The model under review builds one solid part; all positions refer to its coordinate system, in mm. Face numbers are marked on the shaded views. A direction names the side the tool comes from. Round coordinates to 2 decimals unless told otherwise and drop trailing zeros. Write each loop counter-clockwise with the first axis right and the second up, starting at its lowest first coordinate (ties: lowest second). Pieces come first, ordered by that corner, then holes.
Item 1: Add section B-B (z = 153). Give the boundary of the cut face in (x, y) (3 decimals), plus the area to 4 significant figures.
Item 2: Clearance check with flat-ended pins moving along their axes: pin 1 Ø1.2 at (x, z) = (4, 10) entering from +Y (3 decimals); pin 2 Ø4 at (x, z) = (-3, 182) entering from +Y (3 decimals); pin 3 Ø10 at (x, z) = (4, 85) entering from -Y (3 decimals). State where each tip first meets the part, or that it passes through.
Item 3: Add section A-A (x = 0.5). Give the boundary of the cut face in (y, z) (3 decimals), plus the area to 3 significant figures.
Item 4: To check wall thickness, follow L1, parallel to Y at x = 14.75, z = 3.5 (3 decimals); L2, parallel to Z at x = 11, y = 9.5; L3, parallel to X at y = -9.65, z = 3.5. State the ranges of each line that lie inside material, in increasing order.
Item 5: Machinability: for the marked faces 1, 2, 3, 4 and 5, which of the approach directions +Z, -Z, +X, -X, +Y, -Y give a long, thin tool a straight path to every point of the face, cutting with its end or side? Answer none if there is none.
Autodesk Inventor part; units mm, degrees
ref_plane "YZ Plane" through (0, 0, 0) normal (1, 0, 0) x (0, 1, 0)
ref_plane "XZ Plane" through (0, 0, 0) normal (0, 1, 0) x (-1, 0, 0)
ref_plane "XY Plane" through (0, 0, 0) normal (0, 0, 1) x (1, 0, 0)
sketch "Sketch8" plane through (0, 0, 0) normal (0, 0, 1) x (1, 0, 0)
  line L0 (-18.5, -12.375) -> (18.5, -12.375)
  line L1 (18.5, -12.375) -> (18.5, 12.375)
  line L2 (18.5, 12.375) -> (-18.5, 12.375)
  line L3 (-18.5, 12.375) -> (-18.5, -12.375)
  line L4 (-18.5, -12.375) -> (18.5, 12.375) construction
  line L5 (18.5, -12.375) -> (-18.5, 12.375) construction
  point P0 (0, 0)
  dimension "d43" = 37
  dimension "d44" = 24.75
extrude "Extrusion6" add sketch "Sketch8" along normal blind 7
sketch "Sketch9" plane through (0, 0, 7) normal (0, 0, 1) x (1, 0, 0)
  line L0 (-17, -10.875) -> (17, -10.875)
  line L1 (17, -10.875) -> (17, 10.875)
  line L2 (17, 10.875) -> (-17, 10.875)
  line L3 (-17, 10.875) -> (-17, -10.875)
  line L4 (-17, -10.875) -> (17, 10.875) construction
  line L5 (17, -10.875) -> (-17, 10.875) construction
  line L6 (18.5, 12.375) -> (-18.5, 12.375)
  line L7 (18.5, -12.375) -> (18.5, 12.375)
  point P0 (0, 0)
  dimension "d49" = 1.5
  dimension "d50" = 1.5
extrude "Extrusion7" add sketch "Sketch9" along normal blind 184.3
sketch "Sketch10" plane through (18.5, -12.375, 0) normal (1, 0, 0) x (0, 0, -1)
  circle A0 centre (-3.5, 21.325) radius 1.5
  line L0 (0, 0) -> (0, 24.75)
  line L1 (0, 24.75) -> (-7, 24.75)
  point P0 (0, 12.375)
  dimension "d53" = 3
  dimension "d56" = 3.425
  dimension "d57" = 3.5
hole "Hole1" at (18.5, 8.95, 3.5) direction (-1, 0, 0) diameter 3 depth 5 tip angle 118
mirror "Mirror1" about plane through (0, 0, 0) normal (0, 1, 0) of "Hole1"
mirror "Mirror2" about plane through (0, 0, 0) normal (1, 0, 0) of "Hole1", "Mirror1"
sketch "Sketch11" plane through (-18.5, -12.375, 0) normal (0, -1, 0) x (1, 0, 0)
  line L0 (18.5, 0) -> (18.5, 7)
  line L1 (37, 7) -> (0, 7)
  line L2 (18.5, 3.5) -> (0, 3.5)
  line L3 (0, 0) -> (0, 7)
  circle A0 centre (9.25, 3.5) radius 1.5
  dimension "d66" = 3
hole "Hole2" at (-9.25, -12.375, 3.5) direction (0, 1, 0) diameter 3 depth 5 tip angle 118
mirror "Mirror3" about plane through (0, 0, 0) normal (1, 0, 0) of "Hole2"
sketch "Sketch12" plane through (0, 0, 191.3) normal (0, 0, 1) x (1, 0, 0)
  circle A0 centre (6.8, 0) radius 1.5
  line L0 (17, -10.875) -> (17, 10.875)
  line L1 (17, 10.875) -> (-17, 10.875)
  point P0 (0, 0)
  dimension "d74" = 3
  dimension "d75" = 10.2
  dimension "d76" = 10.875
hole "Hole3" at (6.8, 0, 191.3) direction (0, 0, -1) diameter 3 depth 5 tip angle 118
mirror "Mirror4" about plane through (0, 0, 0) normal (1, 0, 0) of "Hole3"
sketch "Sketch13" plane through (-17, -10.875, 7) normal (-1, 0, 0) x (0, 0, 1)
  line L0 (0, 21.75) -> (4.1, 21.75)
  line L1 (0, 21.75) -> (184.3, 21.75)
  line L2 (4.1, 21.75) -> (4.1, 0)
  line L3 (0, 0) -> (184.3, 0)
  line L4 (4.1, 21.75) -> (12.1, 21.75)
  line L5 (0, 21.75) -> (184.3, 21.75)
  line L6 (12.1, 21.75) -> (12.1, 0)
  line L7 (12.1, 0) -> (4.1, 0)
  point P0 (-7, 10.875)
  dimension "d84" = 4.1
  dimension "d85" = 90
  dimension "d86" = 8
  dimension "d87" = 90
extrude "Extrusion8" cut sketch "Sketch13" against normal blind 2
mirror "Mirror5" about plane through (0, 0, 0) normal (1, 0, 0) of "Extrusion8"
sketch "Sketch14" plane through (-17, 10.875, 7) normal (0, 1, 0) x (1, 0, 0)
  line L0 (34, -4.1) -> (32, -4.1)
  line L1 (2, -4.1) -> (2, -12.1)
  line L2 (32, -4.1) -> (2, -4.1)
  line L3 (2, -4.1) -> (2, -12.1)
  line L4 (2, -12.1) -> (32, -12.1)
  line L5 (32, -12.1) -> (32, -4.1)
  point P0 (17, 7)
extrude "Extrusion9" cut sketch "Sketch14" against normal blind 2
mirror "Mirror6" about plane through (0, 0, 0) normal (0, 1, 0) of "Extrusion9"
ref_plane "Work Plane4" through (0, 0, 99.15) normal (0, 0, 1) x (1, 0, 0)
mirror "Mirror7" about plane through (0, 0, 99.15) normal (0, 0, 1) of "Extrusion9", "Extrusion8", "Mirror5", "Mirror6"
properties part number "Mold"
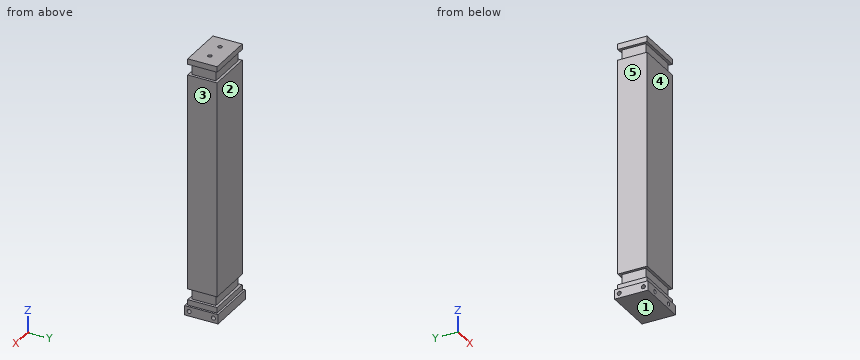
Numbers:
1. outline: (-17, -10.875) - (17, -10.875) - (17, 10.875) - (-17, 10.875) - close
1. area: 739.5 mm2
2. pin 1: stops at y = 10.875
2. pin 2: stops at y = 8.875
2. pin 3: stops at y = -10.875
3. outline: (-12.375, 0) - (12.375, 0) - (12.375, 7) - (10.875, 7) - (10.875, 11.1) - (8.875, 11.1) - (8.875, 19.1) - (10.875, 19.1) - (10.875, 179.2) - (8.875, 179.2) - (8.875, 187.2) - (10.875, 187.2) - (10.875, 191.3) - (-10.875, 191.3) - (-10.875, 187.2) - (-8.875, 187.2) - (-8.875, 179.2) - (-10.875, 179.2) - (-10.875, 19.1) - (-8.875, 19.1) - (-8.875, 11.1) - (-10.875, 11.1) - (-10.875, 7) - (-12.375, 7) - close
3. area: 4,120 mm2
4. L1: y = -12.375 to -10.45, -7.45 to 7.45, 10.45 to 12.375
4. L2: z = 0 to 11.1, 19.1 to 179.2, 187.2 to 191.3
4. L3: x = -13.02 to -10.75, -7.75 to 7.75, 10.75 to 13.02
5. face 1: -Z, +X, -X, +Y, -Y
5. face 2: +Z, +X, -X, +Y
5. face 3: +Z, +X, +Y, -Y
5. face 4: +Z, +X, -X, -Y
5. face 5: +Z, -X, +Y, -Y
